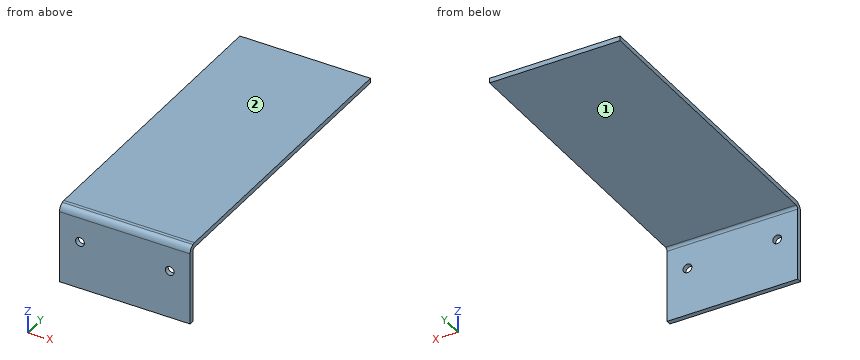
from build123d import *

# Parameters (mm, degrees)
SKETCH1_W              = 43.69375
SKETCH1_H              = 126.6
SKETCH1_R              = 1.4732
BASE_FLANGE1_DEPTH     = 1.6002
SKETCHED_BEND1_DEPTH   = 43.69375
SKETCHED_BEND1_2_DEPTH = 43.69375


# Read off the part's stored shape, not the designer's step: Sketched Bend1
# Sheet-metal steps are written as plain solids
with BuildPart() as part:
    # Sketch1 → Base-Flange1 (new body)
    with BuildSketch(Plane(origin=(0, 0, 0), x_dir=(1, 0, 0), z_dir=(0, 1, 0))):
        with Locations((21.846875, -63.3)):
            Rectangle(SKETCH1_W, SKETCH1_H)
        with Locations(Location((6.846875, -16.01, 0), (0, 0, 270))):
            Circle(SKETCH1_R, mode=Mode.SUBTRACT)
        with Locations(Location((36.846875, -16.01, 0), (0, 0, 270))):
            Circle(SKETCH1_R, mode=Mode.SUBTRACT)
    extrude(amount=-BASE_FLANGE1_DEPTH)

    # Sketched Bend1 outline → Sketched Bend1 (cut)
    with BuildSketch(Plane.YZ):
        with BuildLine():
            ThreePointArc((-1.6002, 24.173927493), (-1.16148963, 25.585171243), (0, 26.49896419))
            Line((0, 26.49896419), (0, 126.6))
            Line((0, 126.6), (-1.6002, 126.6))
            Line((-1.6002, 126.6), (-1.6002, 24.173927493))
        make_face()
    extrude(amount=SKETCHED_BEND1_DEPTH, mode=Mode.SUBTRACT)

    # Sketched Bend1 2 outline → Sketched Bend1 2 (add)
    with BuildSketch(Plane.YZ):
        with BuildLine():
            ThreePointArc((0, 24.173927493), (0.260382071, 24.802545421), (0.889, 25.062927493))
            Line((0.889, 25.062927493), (100.862927493, 25.062927493))
            Line((100.862927493, 25.062927493), (100.862927493, 26.663127493))
            Line((100.862927493, 26.663127493), (0.889, 26.663127493))
            ThreePointArc((0.889, 26.663127493), (0.436984903, 26.62174264), (0, 26.49896419))
            Line((0, 26.49896419), (0, 24.173927493))
        make_face()
    extrude(amount=SKETCHED_BEND1_2_DEPTH)


solid = part.part
Design review of the part built by this model. Coordinates are the model's own, in mm. Face numbers are marked on the shaded views. A direction names the side the tool comes from. Round coordinates to 2 decimals unless told otherwise and drop trailing zeros. Write each loop counter-clockwise with the first axis right and the second up, starting at its lowest first coordinate (ties: lowest second). Pieces come first, ordered by that corner, then holes. Notation, with made-up numbers: M 86,2 L 123,2 A23 cw 123,21 Z; hole C 45,44.5 d3. An arc over 180 degrees is marked long. One line per item, written item: value. Start each with the question number.
1. To check wall thickness, follow probe 1 along X at (y, z) = (-1.2, 16.01); probe 2 along Y at (x, z) = (22.5, 19.5); probe 3 along Z at (x, y) = (13, 55.5). State the ranges of each line that lie inside material, in increasing order. Write a range as from..to.
2. For the marked faces 1 and 2, list the 3-axis set-ups (+Z, -Z, +X, -X, +Y, -Y) from which the entire face can be reached by the end or side of a thin tool; tool diameter is ignored.
3. Clearance check with flat-ended pins moving along their axes: P1, Ø1, axis at x = 30.5, y = 81.5, coming from the -Z side; P2, Ø1, axis at x = 12.5, z = 3.5, coming from the +Y side. State where each tip first meets the part, or that it passes through.
4. Take a section at B-B on x = 16.5. State the section outline as (y, z) points, then the cut area to 3 significant figures.
5. Take a section at C-C on y = 80.5. State the section outline as (x, z) points.
6. Take a section at A-A on z = 16.01. State the section outline as (x, y) points, then the cut area to 3 significant figures.
Computed:
1. probe 1: x = 0..5.37, 8.32..35.37, 38.32..43.69
1. probe 2: y = -1.6..0
1. probe 3: z = 25.06..26.66
2. face 1: -Z, +X, -X, +Y
2. face 2: +Z, +X, -X, +Y, -Y
3. P1: stops at z = 25.06
3. P2: stops at y = 0
4. outline: M -1.6,0 L 0,0 L 0,24.17 A0.89 cw 0.89,25.06 L 100.86,25.06 L 100.86,26.66 L 0.89,26.66 A2.49 ccw -1.6,24.17 Z
4. area: 203 mm²
5. outline: M 0,25.06 L 43.69,25.06 L 43.69,26.66 L 0,26.66 Z
6. outline: M 0,-1.6 L 5.37,-1.6 L 5.37,0 L 0,0 Z; M 8.32,-1.6 L 35.37,-1.6 L 35.37,0 L 8.32,0 Z; M 38.32,-1.6 L 43.69,-1.6 L 43.69,0 L 38.32,0 Z
6. area: 60.5 mm²
